from build123d import *

# Parameters (mm, degrees)
SKETCH_W        = 111.025
SKETCH_H        = 59
SKETCH_R        = 2.5
SKETCH_R_2      = 2
PAD_DEPTH       = 7.5
SKETCH001_W     = 42.5
SKETCH001_H     = 59
POCKET_DEPTH    = 2.5
SKETCH002_W     = 81.025
SKETCH002_H     = 20.325
SKETCH002_W_2   = 43.6
SKETCH002_H_2   = 23.675
SKETCH002_W_3   = 27.425
POCKET001_DEPTH = 7.501
FILLET_R        = 5


with BuildPart() as part:
    # Sketch → Pad (new body)
    with BuildSketch(Plane.XY):
        with Locations((51.1625, 29.5)):
            Rectangle(SKETCH_W, SKETCH_H)
        with Locations((3.15, 22.85)):
            Circle(SKETCH_R, mode=Mode.SUBTRACT)
        with Locations((3.15, 10.6)):
            Circle(SKETCH_R, mode=Mode.SUBTRACT)
        with Locations((27.25, 33.675)):
            Circle(SKETCH_R, mode=Mode.SUBTRACT)
        with Locations((43.075, 19.825)):
            Circle(SKETCH_R_2, mode=Mode.SUBTRACT)
        with Locations((99.175, 19.825)):
            Circle(SKETCH_R_2, mode=Mode.SUBTRACT)
        with Locations((43.075, 4.025)):
            Circle(SKETCH_R_2, mode=Mode.SUBTRACT)
        with Locations((99.175, 4.025)):
            Circle(SKETCH_R_2, mode=Mode.SUBTRACT)
        with Locations((3.15, 50)):
            Circle(SKETCH_R, mode=Mode.SUBTRACT)
        with Locations((99.175, 50)):
            Circle(SKETCH_R, mode=Mode.SUBTRACT)
    extrude(amount=PAD_DEPTH)

    # Sketch001 → Pocket (cut)
    with BuildSketch(Plane.XY.offset(7.5)):
        with Locations((16.9, 29.5)):
            Rectangle(SKETCH001_W, SKETCH001_H)
    extrude(amount=-POCKET_DEPTH, mode=Mode.SUBTRACT)

    # Sketch002 → Pocket001 (cut, through all)
    with BuildSketch(Plane.XY.offset(7.5)):
        with Locations((51.1625, 48.8375)):
            Rectangle(SKETCH002_W, SKETCH002_H)
        with Locations((69.875, 16.8375)):
            Rectangle(SKETCH002_W_2, SKETCH002_H_2)
        with Locations((24.3625, 16.8375)):
            Rectangle(SKETCH002_W_3, SKETCH002_H_2)
    extrude(amount=-POCKET001_DEPTH, mode=Mode.SUBTRACT)

    # Fillet
    fillet_edges = [part.edges().sort_by_distance(p)[0] for p in [
        (106.675, 59, 3.75),
        (91.675, 59, 3.75),
        (91.675, 38.675, 3.75),
        (91.675, 28.675, 3.75),
        (91.675, 5, 3.75),
        (106.675, 0, 3.75),
        (48.075, 5, 3.75),
        (48.075, 28.675, 3.75),
        (38.075, 28.675, 2.5),
        (38.075, 5, 2.5),
        (38.15, 0, 6.25),
        (38.15, 38.675, 6.25),
        (10.65, 5, 2.5),
        (10.65, 28.675, 2.5),
        (10.65, 38.675, 2.5),
        (10.65, 59, 2.5),
        (-4.35, 59, 2.5),
        (-4.35, 0, 2.5),
    ]]
    fillet(fillet_edges, radius=FILLET_R)


solid = part.part
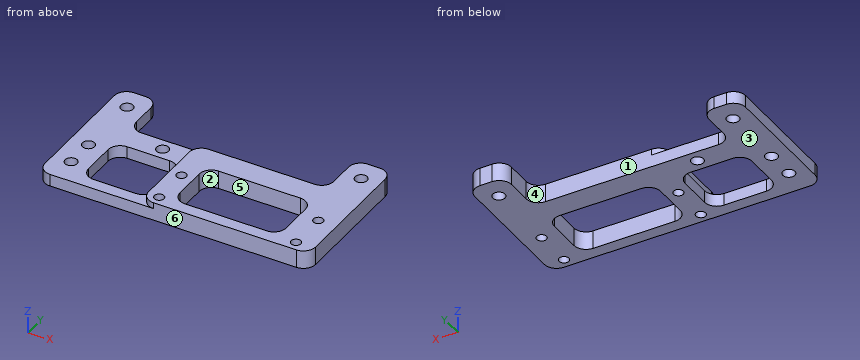
For this review, take the finished solid that the model builds, in its own axes (mm). Face numbers are marked on the shaded views. A direction names the side the tool comes from. Round coordinates to 2 decimals unless told otherwise and drop trailing zeros. Loops run counter-clockwise (first coordinate to the right, second up) from the corner with the lowest first, then second, coordinate; pieces in that order, holes last. Notation, with made-up numbers: (3.5, -25.75) - (20.5, -25.75) arc R22 cw to (20.5, 1.25) - close; hole circle Ø8 at (13.5, 24). An arc over 180 degrees is marked (long way). One line per item, written item: value. Start each with the question number.
Item 1: The part is to be moulded in two halves that separate along Y. For the marked faces 1, 2 and 3, say which applies: +Y half, -Y half, draft (parallel to the pull), parting line (faces both ways), or undercut.
Item 2: For the marked faces 4, 5 and 6, list the 3-axis set-ups (+Z, -Z, +X, -X, +Y, -Y) from which the entire face can be reached by the end or side of a thin tool; tool diameter is ignored.
Item 3: Take a section at D-D (x = 27.25). Give the boundary of the cut face in (y, z) (3 decimals).
Item 4: Take a section at B-B (x = 3.15). Give the boundary of the cut face in (y, z).
Item 5: Clearance check with flat-ended pins moving along their axes: pin 1 Ø6 at (x, y) = (3.15, 22.85) entering from +Z; pin 2 Ø2 at (y, z) = (22, 6.5) entering from -X. State where each tip first meets the part, or that it passes through.
Item 6: For L1, parallel to X at y = 16, z = 2 (3 decimals); L2, parallel to Y at x = 27, z = 0.5 (3 decimals); L3, parallel to X at y = 43.5, z = 1 (3 decimals), list the stretches that pass through material, from the lowest coordinate up.
Item 7: Take a section at C-C (x = 74.5). Give the boundary of the cut face in (y, z) (3 decimals), plus the area to 4 significant figures.
Item 8: Take a section at A-A (y = 50). Give the boundary of the cut face in (x, z) (3 decimals), plus the area to 3 significant figures.
Answer below:
1. face 1: +Y half
1. face 2: undercut
1. face 3: draft
2. face 4: +Z, -Z, +Y
2. face 5: +Z, -Z
2. face 6: +Z, -Z, +X, -X, -Y
3. outline: (0, 0) - (5, 0) - (5, 5) - (0, 5) - close; (28.675, 0) - (31.175, 0) - (31.175, 5) - (28.675, 5) - close; (36.175, 0) - (38.675, 0) - (38.675, 5) - (36.175, 5) - close
4. outline: (0, 0) - (8.1, 0) - (8.1, 5) - (0, 5) - close; (13.1, 0) - (20.35, 0) - (20.35, 5) - (13.1, 5) - close; (25.35, 0) - (47.5, 0) - (47.5, 5) - (25.35, 5) - close; (52.5, 0) - (59, 0) - (59, 5) - (52.5, 5) - close
5. pin 1: stops at z = 5
5. pin 2: stops at x = 38.15
6. L1: x = -4.35 to 10.65, 38.075 to 48.075, 91.675 to 106.675
6. L2: y = 0 to 5, 28.675 to 31.188, 36.162 to 38.675
6. L3: x = -4.35 to 10.653, 91.672 to 106.675
7. outline: (0, 0) - (5, 0) - (5, 7.5) - (0, 7.5) - close; (28.675, 0) - (38.675, 0) - (38.675, 7.5) - (28.675, 7.5) - close
7. area: 112.5 mm2
8. outline: (-4.35, 0) - (0.65, 0) - (0.65, 5) - (-4.35, 5) - close; (5.65, 0) - (10.65, 0) - (10.65, 5) - (5.65, 5) - close; (91.675, 0) - (96.675, 0) - (96.675, 7.5) - (91.675, 7.5) - close; (101.675, 0) - (106.675, 0) - (106.675, 7.5) - (101.675, 7.5) - close
8. area: 125 mm2
